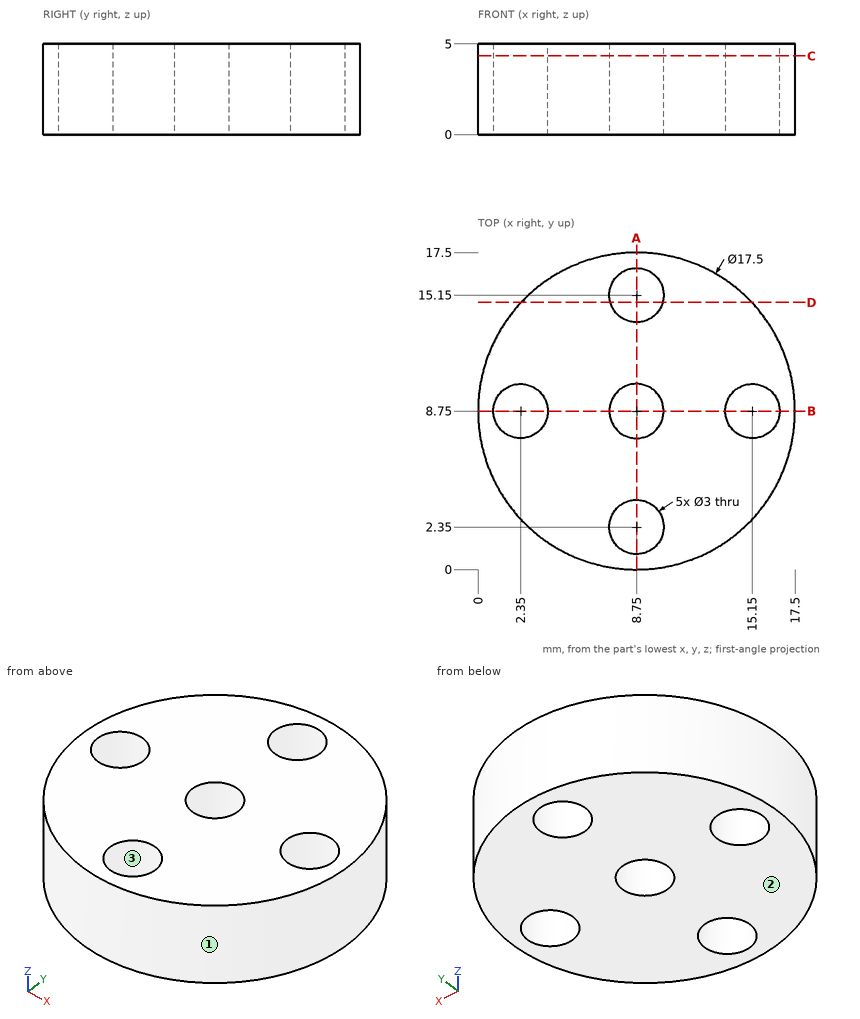
Here's the drawing with two shaded views (mm, measured from the low corner). I have some questions. Round coordinates to 2 decimals unless told otherwise and drop trailing zeros. Loops run counter-clockwise (first coordinate to the right, second up) from the corner with the lowest first, then second, coordinate; pieces in that order, holes last. Notation, with made-up numbers: M -33,78 L 5,78 A26 cw 5,100 Z; hole C 86.25,21.25 d3. An arc over 180 degrees is marked long. Answer as a JSON object with one key per item and string values. Group by question number.
Q1. Imagine slicing it at D-D, the plane y = 14.75. Please give me the cut outline in (x, z), then the cut area to 3 significant figures.
Q2. Imagine slicing it at C-C, the plane z = 4.35. Please give me the cut outline in (x, y), then the cut area to 3 significant figures.
Q3. Will these pins go through, and if not, where does the flat tip stop? pin 1 (5 mm diameter, centred on x = 8.75, y = 2.35, fed in from +Z); pin 2 (3 mm diameter, centred on y = 15.5, z = 4, fed in from +X); pin 3 (1 mm diameter, centred on x = 11.5, z = 1, fed in from -Y); pin 4 (1.5 mm diameter, centred on x = 15, z = 3.5, fed in from +Y).
Q4. We'd pull the mould along Y, two halves only. Please class the marked faces 1, 2 and 3: +Y half, -Y half, draft (parallel to the pull), parting line (faces both ways), or undercut.
Q5. Imagine slicing it at A-A, the plane x = 8.75. Please give me the cut outline in (y, z), then the cut area to 3 significant figures.
Q6. Please list where these lines run through material, in increasing order: L1, parallel to Y at x = 8.75, z = 1.7; L2, parallel to X at y = 10, z = 0.9; L3, parallel to X at y = 3.5, z = 3.85.
Findings:
{
 "1": {"outline": "M 2.38,0 L 7.3,0 L 7.3,5 L 2.38,5 Z; M 10.2,0 L 15.12,0 L 15.12,5 L 10.2,5 Z", "area": "49.2 mm2"},
 "2": {"outline": "C 8.75,8.75 d17.5; hole C 2.35,8.75 d3; hole C 8.75,2.35 d3; hole C 8.75,8.75 d3; hole C 8.75,15.15 d3; hole C 15.15,8.75 d3", "area": "205 mm2"},
 "3": {"pin 1": "stops at z = 5", "pin 2": "stops at x = 15.75", "pin 3": "stops at y = 0.29", "pin 4": "stops at y = 15.56"},
 "4": {"face 1": "parting line", "face 2": "draft", "face 3": "undercut"},
 "5": {"outline": "M 0,0 L 0.85,0 L 0.85,5 L 0,5 Z; M 3.85,0 L 7.25,0 L 7.25,5 L 3.85,5 Z; M 10.25,0 L 13.65,0 L 13.65,5 L 10.25,5 Z; M 16.65,0 L 17.5,0 L 17.5,5 L 16.65,5 Z", "area": "42.5 mm2"},
 "6": {"L1": "y = 0 to 0.85, 3.85 to 7.25, 10.25 to 13.65, 16.65 to 17.5", "L2": "x = 0.09 to 1.52, 3.18 to 7.92, 9.58 to 14.32, 15.98 to 17.41", "L3": "x = 1.75 to 7.79, 9.71 to 15.75"}
}
